Could you check a few things on this model? Use its own coordinates, in mm. A direction names the side the tool comes from. Coordinates: 2 decimals unless noted, no trailing zeros. Write each loop counter-clockwise with the first axis right and the second up, starting at its lowest first coordinate (ties: lowest second). Pieces come first, ordered by that corner, then holes.
Item 1: I want a section at B-B on z = 50.8. Please give me the cut outline in (x, y) (3 decimals).
Item 2: If I drill on probe 1 along X at (y, z) = (2.3, -50.8); probe 2 along X at (y, z) = (25.5, 21); probe 3 along Z at (x, y) = (-1, 17.75) (3 decimals), over which ranges is the centre line in solid material (lowest first)?
Item 3: I want a section at D-D on x = -34.5. Please give me the cut outline in (y, z).
Item 4: I want a section at A-A on y = 16.25. Please give me the cut outline in (x, z) (3 decimals).
Item 5: Which directions (+Z, -Z, +X, -X, +Y, -Y) give clear straight access to the entire face, cutting with the end or side of a thin tool? Please do faces 1 (the flat face through (12.7, 2, -52)), 2 (the flat face through (-12.7, 2, -52)), 3 (the flat face through (-12.7, 2, 52)), 4 (the flat face through (12.7, 17, 21)), 5 (the flat face through (12.7, 2, 52)).
Item 6: For P1, Ø3.5, axis at y = 2, z = 53, coming from the -X side; P2, Ø6, axis at y = 6.5, z = -23.5, coming from the -X side; P3, Ø3, axis at x = 18, z = 9, coming from the +Y side, each with a flat end and sliding along its axis, tell me the tip position at first contact or that it passes through.
Item 7: Thinking about a two-plate mould opening in Z: for faces 6 (the cylindrical face through (-23.183, 16.994, -30.235)), 7 (the flat face through (0, 3.175, 55)), 8 (the cylindrical face through (-14.002, 1.565, -43.682)), which applies, +Z half, -Z half, draft (parallel to the pull), parting line (faces both ways), or undercut?
Item 8: I want a section at C-C on x = 0. Please give me the cut outline in (y, z) (3 decimals).
from build123d import *

# Parameters (mm, degrees)
SKETCH2_R           = 44.45
SKETCH2_R_2         = 38.1
BOSS_EXTRUDE1_DEPTH = 6.35
SKETCH2_3_R         = 44.45
SKETCH2_3_R_2       = 38.1
BOSS_EXTRUDE2_DEPTH = 27.94
SKETCH3_R           = 31.75
BOSS_EXTRUDE4_DEPTH = 21.59
CUT_EXTRUDE1_START  = -1.27
SKETCH4_R           = 2
CUT_EXTRUDE1_DEPTH  = 1.27
CUT_EXTRUDE2_START  = -8.89
SKETCH4_3_R         = 2
CUT_EXTRUDE2_DEPTH  = 8.89
SKETCH5_W           = 25.4
SKETCH5_H           = 25.4
BOSS_EXTRUDE6_DEPTH = 3.175
FILLET1_R           = 7.62
SKETCH7_R           = 1.75
CUT_EXTRUDE3_DEPTH  = 11.43
SKETCH8_W           = 25.4
SKETCH8_H           = 9.525
CUT_EXTRUDE4_DEPTH  = 21.59


with BuildPart() as part:
    # Sketch2 → Boss-Extrude1 (new body)
    # profile 1 of 2: a face of its own
    with BuildSketch(Plane(origin=(0, 0, 0), x_dir=(1, 0, 0), z_dir=(0, 1, 0))):
        with Locations(Location((0, 0, 0), (0, 0, 270))):
            Circle(SKETCH2_R)
        Circle(SKETCH2_R_2, mode=Mode.SUBTRACT)
    # profile 2 of 2: a face of its own
    with BuildSketch(Plane(origin=(0, 0, 0), x_dir=(1, 0, 0), z_dir=(0, 1, 0))):
        Circle(SKETCH2_R_2)
    extrude(amount=BOSS_EXTRUDE1_DEPTH)

    # Sketch2<3> → Boss-Extrude2 (add)
    with BuildSketch(Plane(origin=(0, 0, 0), x_dir=(1, 0, 0), z_dir=(0, 1, 0))):
        with Locations(Location((0, 0, 0), (0, 0, 270))):
            Circle(SKETCH2_3_R)
        with Locations(Location((0, 0, 0), (0, 0, 270))):
            Circle(SKETCH2_3_R_2, mode=Mode.SUBTRACT)
    extrude(amount=BOSS_EXTRUDE2_DEPTH)

    # Sketch3 → Boss-Extrude4 (add)
    # profile 1 of 3: a face of its own
    with BuildSketch(Plane(origin=(0, 6.35, 0), x_dir=(1, 0, 0), z_dir=(0, 1, 0))):
        with Locations(Location((0, 0, 0), (0, 0, 270))):
            Circle(SKETCH3_R)
        with BuildLine():
            ThreePointArc((17.528088934, -11.500057344), (21.028088934, -8.000057344), (17.528088934, -4.500057344))
            Line((17.528088934, -4.500057344), (14.019310816, -4.500057344))
            ThreePointArc((14.019310816, -4.500057344), (0, 6.449547348), (-14.019310816, -4.500057344))
            Line((-14.019310816, -4.500057344), (-17.471911066, -4.500057344))
            ThreePointArc((-17.471911066, -4.500057344), (-20.971911066, -8.000057344), (-17.471911066, -11.500057344))
            Line((-17.471911066, -11.500057344), (-14.019310816, -11.500057344))
            ThreePointArc((-14.019310816, -11.500057344), (0, -22.010555024), (14.019310816, -11.500057344))
            Line((14.019310816, -11.500057344), (17.528088934, -11.500057344))
        make_face(mode=Mode.SUBTRACT)
    # profile 2 of 3: a face of its own
    with BuildSketch(Plane(origin=(0, 6.35, 0), x_dir=(1, 0, 0), z_dir=(0, 1, 0))):
        with BuildLine():
            ThreePointArc((-14.019310816, -4.500057344), (-14.449604692, -8.000057344), (-14.019310816, -11.500057344))
            Line((-14.019310816, -11.500057344), (-17.471911066, -11.500057344))
            ThreePointArc((-17.471911066, -11.500057344), (-20.971911066, -8.000057344), (-17.471911066, -4.500057344))
            Line((-17.471911066, -4.500057344), (-14.019310816, -4.500057344))
        make_face()
    # profile 3 of 3: a face of its own
    with BuildSketch(Plane(origin=(0, 6.35, 0), x_dir=(1, 0, 0), z_dir=(0, 1, 0))):
        with BuildLine():
            Line((17.528088934, -4.500057344), (14.019310816, -4.500057344))
            ThreePointArc((14.019310816, -4.500057344), (14.449604692, -8.000057344), (14.019310816, -11.500057344))
            Line((14.019310816, -11.500057344), (17.528088934, -11.500057344))
            ThreePointArc((17.528088934, -11.500057344), (21.028088934, -8.000057344), (17.528088934, -4.500057344))
        make_face()
    extrude(amount=BOSS_EXTRUDE4_DEPTH)

    # Sketch4 → Cut-Extrude1 (cut)
    # profile 1 of 2: a face of its own
    with BuildSketch(Plane(origin=(0, 27.94, 0), x_dir=(1, 0, 0), z_dir=(0, 1, 0)).offset(CUT_EXTRUDE1_START)):
        with BuildLine():
            Line((17.631328518, -4.762679984), (14.082274801, -4.762679984))
            ThreePointArc((14.082274801, -4.762679984), (14.448973734, -8.135089853), (14.019310816, -11.500057344))
            ThreePointArc((14.019310816, -11.500057344), (13.980234208, -11.631555081), (13.939924214, -11.762679984))
            Line((13.939924214, -11.762679984), (17.631328518, -11.762679984))
            ThreePointArc((17.631328518, -11.762679984), (21.131328518, -8.262679984), (17.631328518, -4.762679984))
        make_face()
        with Locations(Location((17.631328518, -8.262679984, 0), (0, 0, 270))):
            Circle(SKETCH4_R, mode=Mode.SUBTRACT)
    # profile 2 of 2: a face of its own
    with BuildSketch(Plane(origin=(0, 27.94, 0), x_dir=(1, 0, 0), z_dir=(0, 1, 0)).offset(CUT_EXTRUDE1_START)):
        with BuildLine():
            ThreePointArc((-14.019310816, -11.500057344), (-14.448973734, -8.135089853), (-14.082274801, -4.762679984))
            Line((-14.082274801, -4.762679984), (-17.368671482, -4.762679984))
            ThreePointArc((-17.368671482, -4.762679984), (-20.868671482, -8.262679984), (-17.368671482, -11.762679984))
            Line((-17.368671482, -11.762679984), (-13.939924214, -11.762679984))
            ThreePointArc((-13.939924214, -11.762679984), (-13.980234208, -11.631555081), (-14.019310816, -11.500057344))
        make_face()
        with Locations(Location((-17.368671482, -8.262679984, 0), (0, 0, 270))):
            Circle(SKETCH4_R, mode=Mode.SUBTRACT)
    extrude(amount=CUT_EXTRUDE1_DEPTH, mode=Mode.SUBTRACT)

    # Sketch4<3> → Cut-Extrude2 (cut)
    with BuildSketch(Plane(origin=(0, 27.94, 0), x_dir=(1, 0, 0), z_dir=(0, 1, 0)).offset(CUT_EXTRUDE2_START)):
        with Locations(Location((-17.368671482, -8.262679984, 0), (0, 0, 270))):
            Circle(SKETCH4_3_R)
        with Locations(Location((17.631328518, -8.262679984, 0), (0, 0, 270))):
            Circle(SKETCH4_3_R)
    extrude(amount=CUT_EXTRUDE2_DEPTH, mode=Mode.SUBTRACT)

    # Sketch5 → Boss-Extrude6 (add)
    with BuildSketch(Plane.XZ):
        with Locations((0, 50.8)):
            Rectangle(SKETCH5_W, SKETCH5_H)
        with Locations((0, -50.8)):
            Rectangle(SKETCH5_W, SKETCH5_H)
    extrude(amount=-BOSS_EXTRUDE6_DEPTH)

    # Fillet1
    fillet1_edges = [part.edges().sort_by_distance(p)[0] for p in [
        (12.7, 1.5875, 63.5),
        (-12.7, 1.5875, 63.5),
        (12.7, 1.5875, 42.597094971),
        (-12.7, 1.5875, 42.597094971),
        (-12.7, 1.5875, -63.5),
        (12.7, 1.5875, -63.5),
        (-12.7, 1.5875, -42.597094971),
        (12.7, 1.5875, -42.597094971),
    ]]
    fillet(fillet1_edges, radius=FILLET1_R)

    # Sketch7 → Cut-Extrude3 (cut)
    with BuildSketch(Plane(origin=(0, 3.175, 0), x_dir=(1, 0, 0), z_dir=(0, 1, 0))):
        with Locations(Location((0, 50.8, 0), (0, 0, 270))):
            Circle(SKETCH7_R)
        with Locations(Location((0, -50.8, 0), (0, 0, 270))):
            Circle(SKETCH7_R)
    extrude(amount=-CUT_EXTRUDE3_DEPTH, mode=Mode.SUBTRACT)

    # Sketch8 → Cut-Extrude4 (cut)
    with BuildSketch(Plane(origin=(0, 27.94, 0), x_dir=(1, 0, 0), z_dir=(0, 1, 0))):
        with Locations((0, -21.2725)):
            Rectangle(SKETCH8_W, SKETCH8_H)
    extrude(amount=-CUT_EXTRUDE4_DEPTH, mode=Mode.SUBTRACT)


solid = part.part
Response values:
1. outline: (-12.7, 0) - (-1.75, 0) - (-1.75, 3.175) - (-12.7, 3.175) - close; (1.75, 0) - (12.7, 0) - (12.7, 3.175) - (1.75, 3.175) - close
2. probe 1: x = -12.7 to -1.75, 1.75 to 12.7
2. probe 2: x = -39.18 to -31.79, -23.81 to -12.7, 12.7 to 23.81, 31.79 to 39.18
2. probe 3: z = -44.439 to -38.087, -31.734 to -6.415, 26.035 to 31.734, 38.087 to 44.439
3. outline: (0, -28.03) - (27.94, -28.03) - (27.94, -16.17) - (6.35, -16.17) - (6.35, 16.17) - (27.94, 16.17) - (27.94, 28.03) - (0, 28.03) - close
4. outline: circle Ø88.9 at (0, 0); circle Ø63.5 at (0, 0); hole circle Ø76.2 at (0, 0); hole (-14.019, 11.5) arc R14.45 ccw (long way) to (14.019, 11.5) arc R14.605 ccw to (11.42, 16.51) - (12.7, 16.51) - (12.7, 26.035) - (-12.7, 26.035) - (-12.7, 16.51) - (-11.42, 16.51) arc R14.605 ccw to start
5. face 1: -Z, +X, +Y, -Y
5. face 2: -Z, -X, +Y, -Y
5. face 3: +Z, -X, +Y, -Y
5. face 4: +Y
5. face 5: +Z, +X, +Y, -Y
6. P1: stops at x = -12.7
6. P2: stops at x = -39.44
6. P3: stops at y = 26.67
7. face 6: undercut
7. face 7: draft
7. face 8: -Z half
8. outline: (0, -63.5) - (3.175, -63.5) - (3.175, -52.55) - (0, -52.55) - close; (0, -49.05) - (3.175, -49.05) - (3.175, -44.45) - (27.94, -44.45) - (27.94, -38.1) - (6.35, -38.1) - (6.35, -31.75) - (27.94, -31.75) - (27.94, -6.45) - (6.35, -6.45) - (6.35, 26.035) - (27.94, 26.035) - (27.94, 31.75) - (6.35, 31.75) - (6.35, 38.1) - (27.94, 38.1) - (27.94, 44.45) - (3.175, 44.45) - (3.175, 49.05) - (0, 49.05) - close; (0, 52.55) - (3.175, 52.55) - (3.175, 63.5) - (0, 63.5) - close
